Part print with two shaded views. Sizes in mm from the minimum x, y, z corner. Round coordinates to 2 decimals unless told otherwise and drop trailing zeros. Order: outer loops, then holes, each group sorted by start corner. A loop starts at its lowest first (then second) coordinate and runs counter-clockwise, first axis right, second up. Notation, with made-up numbers: (-28, -6) - (-16, -6) arc R17 ccw to (-16, 27) - close; hole circle Ø11 at (52.5, 65.5). An arc over 180 degrees is marked (long way). Use one line per item in the form item = value.
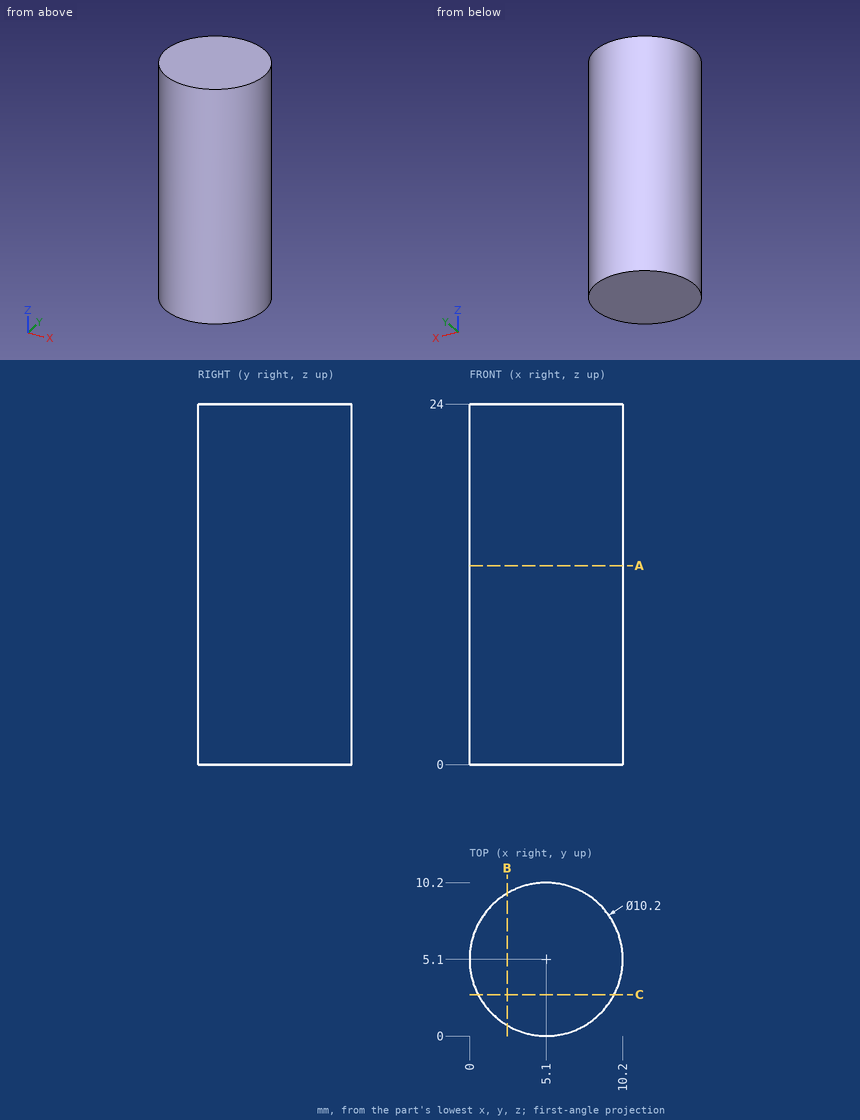
(1) Pin check, flat tips, straight feed: pin 1 (3 mm diameter, centred on x = 8.5, z = 3.5, fed in from +Y); pin 2 (2 mm diameter, centred on y = 8.5, z = 19.5, fed in from -X). Stop position of each tip, or through.
Report:
pin_1 = 9.83
pin_2 = 0.6
(2) Slice it at C-C on y = 2.75. Give the cut face in (x, z).
Report:
outline = (0.57, 0) - (9.63, 0) - (9.63, 24) - (0.57, 24) - close
(3) Probe probe 1 along X at (y, z) = (5, 9.5); probe 2 along Y at (x, z) = (1, 3.75); probe 3 along Y at (x, z) = (8.5, 15.25). List the from-to ranges inside material, lowest first. Write a range as [from, to].
Report:
probe_1 = [0, 10.2]
probe_2 = [2.07, 8.13]
probe_3 = [1.3, 8.9]
(4) Slice it at A-A on z = 13.25. Give the cut face in (x, y).
Report:
outline = circle Ø10.2 at (5.1, 5.1)
(5) Slice it at B-B on x = 2.5. Give the cut face in (y, z), then the cut area to 3 significant figures.
Report:
outline = (0.71, 0) - (9.49, 0) - (9.49, 24) - (0.71, 24) - close
area = 211 mm2
